```python
from build123d import *

# Parameters (mm, degrees)
F1_DEPTH = 101.6
F3_D     = 22.86


# Not quite as in the source:
# - a feature names something its author has since deleted; it is built from what else it names
# - the program builds the solid bodies; features that only make, move or delete a surface that nothing else refers to are left out


with BuildPart() as f1:
    # F0 (on Front) → F1 (new body)
    with BuildSketch(Plane.XZ):
        with BuildLine():
            Line((-132.1375894797, -18.6150499344), (-132.1375894797, -44.0150499344))
            Line((-132.1375894797, -44.0150499344), (-68.6375894797, -44.0150499344))
            ThreePointArc((-68.6375894797, -44.0150499344), (-8.0905175805, 0.345930121), (52.4565543186, -44.0150499344))
            Line((52.4565543186, -44.0150499344), (115.9565543186, -44.0150499344))
            Line((115.9565543186, -44.0150499344), (115.9565543186, -18.6150499344))
            Line((115.9565543186, -18.6150499344), (65.1565543186, -18.6150499344))
            ThreePointArc((65.1565543186, -18.6150499344), (-8.0905175805, 19.9056243635), (-81.3375894797, -18.6150499344))
            Line((-81.3375894797, -18.6150499344), (-132.1375894797, -18.6150499344))
        make_face()
    extrude(amount=F1_DEPTH)

    # F3 (through all)
    with Locations(Plane.XY.offset(-18.6150499344)):
        with Locations((-104.1975894797, -27.5148972869), (-104.1975894797, -73.2348972869)):
            Hole(F3_D / 2)


solid = f1.part
```
For this review, take the finished solid that the model builds, in its own axes (mm). A direction names the side the tool comes from. Give positions to 0.01 mm unless a question says otherwise; leave off trailing zeros. Loops run counter-clockwise (first coordinate to the right, second up) from the corner with the lowest first, then second, coordinate; pieces in that order, holes last. Notation, with made-up numbers: M -10.5,5 L 37.5,5 A24 cw 37.5,44 Z; hole C 21.25,28 d1. An arc over 180 degrees is marked long. One line per item, written item: value. Start each with the question number.
Q1. Clearance check with flat-ended pins moving along their axes: pin 1 Ø8 at (x, y) = (-88.5, -26.5) entering from +Z; pin 2 Ø6 at (x, y) = (12, -79) entering from -Z; pin 3 Ø3 at (y, z) = (-34.5, -6.5) entering from -X. State where each tip first meets the part, or that it passes through.
Q2. Add section D-D (z = -21.5). Give the boundary of the cut face in (x, y), and give its area (3 significant figures).
Q3. Machinability: for faces 1 (the face through (84, -50, -44.015)), 2 (the face through (91, -50, -18.615)), which of the approach directions +Z, -Z, +X, -X, +Y, -Y give a long, thin tool a straight path to every point of the face, cutting with its end or side? Answer none if there is none.
Q4. Add section A-A (z = -36.5). Give the boundary of the cut face in (x, y).
Q5. For L1, parallel to Z at x = -111.5, y = -64; L2, parallel to X at y = -77.5, z = -20; L3, parallel to X at y = -91.5, z = -36, list the stretches that pass through material, from the lowest coordinate up.
Q6. Add section C-C (x = -102). Give the boundary of the cut face in (y, z).
Q7. Add section B-B (y = -50). Give the boundary of the cut face in (x, z), and give its area (3 significant figures).
Q8. Draft analysis for pull direction Z (two halves, no side actions). For faces 3 (the face through (-115.1, -24.08, -31.49)), 4 (the face through (-101, -50, -44.015)), 5 (the face through (-106, -50, -18.615)), state which applies: released by +Z, released by -Z, zero draft, split by the parting line, or undercut.
Reply:
1. pin 1: z = -18.62
1. pin 2: z = -4
1. pin 3: x = -72.77
2. outline: M -132.14,-101.6 L -56.02,-101.6 L -56.02,0 L -132.14,0 Z; M 39.84,-101.6 L 115.96,-101.6 L 115.96,0 L 39.84,0 Z; hole C -104.2,-73.23 d22.86; hole C -104.2,-27.51 d22.86
2. area: 14,600 mm²
3. face 1: -Z, +X, -X, +Y, -Y
3. face 2: +Z, +X, +Y, -Y
4. outline: M -132.14,-101.6 L -65.73,-101.6 L -65.73,0 L -132.14,0 Z; M 49.54,-101.6 L 115.96,-101.6 L 115.96,0 L 49.54,0 Z; hole C -104.2,-73.23 d22.86; hole C -104.2,-27.51 d22.86
5. L1: -44.02 to -18.62
5. L2: -132.14 to -114.8, -93.59 to -54.67, 38.49 to 115.96
5. L3: -132.14 to -65.49, 49.31 to 115.96
6. outline: M -101.6,-44.02 L -84.45,-44.02 L -84.45,-18.62 L -101.6,-18.62 Z; M -62.02,-44.02 L -38.73,-44.02 L -38.73,-18.62 L -62.02,-18.62 Z; M -16.3,-44.02 L 0,-44.02 L 0,-18.62 L -16.3,-18.62 Z
7. outline: M -132.14,-44.02 L -68.64,-44.02 A63.5 cw 52.46,-44.02 L 115.96,-44.02 L 115.96,-18.62 L 65.16,-18.62 A88.9 ccw -81.34,-18.62 L -132.14,-18.62 Z
7. area: 6,320 mm²
8. face 3: zero draft
8. face 4: released by -Z
8. face 5: released by +Z
